from build123d import *

# Parameters (mm, degrees)
BOSS_EXTRUDE1_DEPTH = 45
SKETCH4_R           = 1.35
CUT_EXTRUDE3_DEPTH  = 88.759301296
SKETCH16_W          = 54.601375451
SKETCH16_H          = 80.563035577
CUT_EXTRUDE6_DEPTH  = 86.719849393
SKETCH17_W          = 45
SKETCH17_H          = 36.75
SKETCH17_W_2        = 30
SKETCH17_H_2        = 30
CUT_EXTRUDE7_DEPTH  = 74.310606081
SKETCH18_R          = 1.35
CUT_EXTRUDE8_DEPTH  = 64.93499752
FILLET1_R           = 8.89
SKETCH19_W          = 11
SKETCH19_H          = 11
BOSS_EXTRUDE2_DEPTH = 2.921
SKETCH20_W          = 5
SKETCH20_H          = 5
CUT_EXTRUDE9_DEPTH  = 25
SKETCH26_W          = 32.004
SKETCH26_H          = 43.2054
BOSS_EXTRUDE3_DEPTH = 2.54
SKETCH27_W          = 32.004
SKETCH27_H          = 22.606
BOSS_EXTRUDE4_DEPTH = 11.7475
SKETCH28_R          = 1.2954
CUT_EXTRUDE11_DEPTH = 19.05
CUT_EXTRUDE14_DEPTH = 3.81
SKETCH32_W          = 2.921
SKETCH32_H          = 9.5
BOSS_EXTRUDE5_DEPTH = 10.922
SKETCH33_W          = 11.7475
SKETCH33_H          = 20.574
CUT_EXTRUDE15_DEPTH = 78.55193447
FILLET2_R           = 5.08
FILLET3_R           = 5.08
FILLET4_R           = 7.62
FILLET5_R           = 7.62
FILLET6_R           = 7.62
FILLET7_R           = 2.54
FILLET8_R           = 2.54
FILLET9_R           = 2.54
FILLET10_R          = 2.54
CUT_EXTRUDE16_START = -11.43
SKETCH34_R          = 1.35
CUT_EXTRUDE16_DEPTH = 11.43


with BuildPart() as part:
    # Sketch1 → Boss-Extrude1 (new body)
    with BuildSketch(Plane.XY):
        Polygon((-3.796, -4.492), (-3.796, 57.658), (44.704, 57.658), (44.704, 20.908), (39.704, 20.908), (39.704, 52.658), (1.204, 52.658), (1.204, -4.492), align=None)
    extrude(amount=BOSS_EXTRUDE1_DEPTH)

    # Sketch4 → Cut-Extrude3 (cut, through all)
    with BuildSketch(Plane(origin=(44.704, 0, 0), x_dir=(0, 0, -1), z_dir=(1, 0, 0))):
        with Locations(Location((-22.6336, 47.4432, 0), (0, 0, 90))):
            Circle(SKETCH4_R)
        with Locations(Location((-22.6336, 25.448, 0), (0, 0, 90))):
            Circle(SKETCH4_R)
        with Locations(Location((-11.6341, 36.4435, 0), (0, 0, 90))):
            Circle(SKETCH4_R)
        with Locations(Location((-33.6321, 36.4435, 0), (0, 0, 90))):
            Circle(SKETCH4_R)
    extrude(amount=-CUT_EXTRUDE3_DEPTH, mode=Mode.SUBTRACT)

    # Sketch16 → Cut-Extrude6 (cut, through all)
    with BuildSketch(Plane.XY.offset(45)):
        with Locations((12.403312274, 23.911522997)):
            Rectangle(SKETCH16_W, SKETCH16_H)
    extrude(amount=-CUT_EXTRUDE6_DEPTH, mode=Mode.SUBTRACT)

    # Sketch17 → Cut-Extrude7 (cut, through all)
    with BuildSketch(Plane(origin=(44.704, 0, 0), x_dir=(0, 0, -1), z_dir=(1, 0, 0))):
        with Locations((-22.5, 39.283)):
            Rectangle(SKETCH17_W, SKETCH17_H)
        with Locations((-22.6331, 36.4435)):
            Rectangle(SKETCH17_W_2, SKETCH17_H_2, mode=Mode.SUBTRACT)
    extrude(amount=-CUT_EXTRUDE7_DEPTH, mode=Mode.SUBTRACT)

    # Sketch18 → Cut-Extrude8 (cut, through all)
    with BuildSketch(Plane(origin=(44.704, 0, 0), x_dir=(0, 0, -1), z_dir=(1, 0, 0))):
        with Locations(Location((-14.857193174, 44.222006826, 0), (0, 0, 90))):
            Circle(SKETCH18_R)
        with Locations(Location((-30.410360379, 28.668839621, 0), (0, 0, 90))):
            Circle(SKETCH18_R)
        with Locations(Location((-14.856839621, 28.668839621, 0), (0, 0, 90))):
            Circle(SKETCH18_R)
        with Locations(Location((-30.410360379, 44.222006826, 0), (0, 0, 90))):
            Circle(SKETCH18_R)
    extrude(amount=-CUT_EXTRUDE8_DEPTH, mode=Mode.SUBTRACT)

    # Fillet1
    fillet1_edges = [part.edges().sort_by_distance(p)[0] for p in [
        (42.204, 51.4435, 7.6331),
        (42.204, 51.4435, 37.6331),
        (42.204, 21.4435, 37.6331),
        (42.204, 21.4435, 7.6331),
    ]]
    fillet(fillet1_edges, radius=FILLET1_R)

    # Sketch19 → Boss-Extrude2 (add)
    with BuildSketch(Plane(origin=(44.704, 0, 0), x_dir=(0, 0, -1), z_dir=(1, 0, 0))):
        with Locations((-22.6336, 36.4435)):
            Rectangle(SKETCH19_W, SKETCH19_H)
    extrude(amount=BOSS_EXTRUDE2_DEPTH)

    # Sketch20 → Cut-Extrude9 (cut)
    with BuildSketch(Plane(origin=(47.625, 0, 0), x_dir=(0, 0, -1), z_dir=(1, 0, 0))):
        with Locations((-22.6336, 36.4435)):
            Rectangle(SKETCH20_W, SKETCH20_H)
    extrude(amount=-CUT_EXTRUDE9_DEPTH, mode=Mode.SUBTRACT)

    # Sketch26 → Boss-Extrude3 (add)
    with BuildSketch(Plane(origin=(47.625, 0, 0), x_dir=(0, 0, -1), z_dir=(1, 0, 0))):
        with Locations((-22.6336, 24.202149454)):
            Rectangle(SKETCH26_W, SKETCH26_H)
    extrude(amount=BOSS_EXTRUDE3_DEPTH)

    # Sketch27 → Boss-Extrude4 (add)
    with BuildSketch(Plane(origin=(50.165, 0, 0), x_dir=(0, 0, -1), z_dir=(1, 0, 0))):
        with Locations((-22.6336, 13.902449454)):
            Rectangle(SKETCH27_W, SKETCH27_H)
    extrude(amount=BOSS_EXTRUDE4_DEPTH)

    # Sketch28 → Cut-Extrude11 (cut)
    with BuildSketch(Plane(origin=(61.9125, 0, 0), x_dir=(0, 0, -1), z_dir=(1, 0, 0))):
        with Locations((-9.1208, 21.903449454)):
            Circle(SKETCH28_R)
        with Locations((-9.1208, 5.901449454)):
            Circle(SKETCH28_R)
        with Locations((-36.1464, 5.901449454)):
            Circle(SKETCH28_R)
        with Locations((-36.1464, 21.903449454)):
            Circle(SKETCH28_R)
    extrude(amount=-CUT_EXTRUDE11_DEPTH, mode=Mode.SUBTRACT)

    # Sketch31 → Cut-Extrude14 (cut)
    with BuildSketch(Plane(origin=(50.165, 0, 0), x_dir=(0, 0, -1), z_dir=(1, 0, 0))):
        Polygon((-38.6356, 45.804849454), (-38.6356, 30.9435), (-28.1336, 30.9435), (-28.1336, 41.9435), (-17.1336, 41.9435), (-17.1336, 30.9435), (-6.6316, 30.9435), (-6.6316, 45.804849454), align=None)
    extrude(amount=-CUT_EXTRUDE14_DEPTH, mode=Mode.SUBTRACT)

    # Sketch32 → Boss-Extrude5 (add)
    with BuildSketch(Plane(origin=(0, 0, 17.1336), x_dir=(-1, 0, 0), z_dir=(0, 0, -1))):
        with Locations((-46.1645, 26.1935)):
            Rectangle(SKETCH32_W, SKETCH32_H)
    extrude(amount=-BOSS_EXTRUDE5_DEPTH)

    # Sketch33 → Cut-Extrude15 (cut, through all)
    with BuildSketch(Plane(origin=(0, 25.205449454, 0), x_dir=(1, 0, 0), z_dir=(0, 1, 0))):
        with Locations((56.03875, -22.6336)):
            Rectangle(SKETCH33_W, SKETCH33_H)
    extrude(amount=-CUT_EXTRUDE15_DEPTH, mode=Mode.SUBTRACT)

    # Fillet2
    fillet2_edges = [part.edges().sort_by_distance(p)[0] for p in [
        (50.165, 25.205449454, 35.7781),
    ]]
    fillet(fillet2_edges, radius=FILLET2_R)

    # Fillet3
    fillet3_edges = [part.edges().sort_by_distance(p)[0] for p in [
        (50.165, 25.205449454, 9.4891),
    ]]
    fillet(fillet3_edges, radius=FILLET3_R)

    # Fillet4
    # the kernel refuses this fillet: 7.62 mm, written as the material it adds along each edge
    with BuildSketch(Plane(origin=(47.625, 21.4435, 17.1336), x_dir=(-1, 0, 0), z_dir=(0, 0, 1))) as fillet4_piece_1:
        with BuildLine():
            CenterArc((FILLET4_R, FILLET4_R), FILLET4_R, 180, 90)
            Line((0, FILLET4_R), (0, 0))
            Line((0, 0), (FILLET4_R, 0))
        make_face()
    extrude(amount=10.922)

    # Fillet5
    fillet5_edges = [part.edges().sort_by_distance(p)[0] for p in [
        (48.895, 30.9435, 17.1336),
    ]]
    fillet(fillet5_edges, radius=FILLET5_R)

    # Fillet6
    fillet6_edges = [part.edges().sort_by_distance(p)[0] for p in [
        (48.895, 30.9435, 28.1336),
    ]]
    fillet(fillet6_edges, radius=FILLET6_R)

    # Fillet7
    fillet7_edges = [part.edges().sort_by_distance(p)[0] for p in [
        (47.4345, 41.9435, 28.1336),
    ]]
    fillet(fillet7_edges, radius=FILLET7_R)

    # Fillet8
    fillet8_edges = [part.edges().sort_by_distance(p)[0] for p in [
        (47.4345, 41.9435, 17.1336),
    ]]
    fillet(fillet8_edges, radius=FILLET8_R)

    # Fillet9
    fillet9_edges = [part.edges().sort_by_distance(p)[0] for p in [
        (47.625, 22.3835, 28.0556),
    ]]
    fillet(fillet9_edges, radius=FILLET9_R)

    # Fillet10
    fillet10_edges = [part.edges().sort_by_distance(p)[0] for p in [
        (47.625, 26.1935, 17.1336),
    ]]
    fillet(fillet10_edges, radius=FILLET10_R)

    # Sketch34 → Cut-Extrude16 (cut)
    with BuildSketch(Plane.ZY.offset(-39.704).offset(CUT_EXTRUDE16_START)):
        with Locations(Location((22.6336, 25.448, 0), (0, 0, 90))):
            Circle(SKETCH34_R)
    extrude(amount=CUT_EXTRUDE16_DEPTH, mode=Mode.SUBTRACT)


solid = part.part
Can you work these out from the model? Positions are in its coordinate system, mm. A direction names the side the tool comes from. Give positions to 0.01 mm unless a question says otherwise; leave off trailing zeros. Order: outer loops, then holes, each group sorted by start corner. A loop starts at its lowest first (then second) coordinate and runs counter-clockwise, first axis right, second up. Notation, with made-up numbers: M 79,-34.5 L 85,-34.5 A34 cw 85,1.5 Z; hole C -27,-4 d8. An arc over 180 degrees is marked long. Use one line per item in the form item = value. Start each with the question number.
Item 1: If I drill on line 1 along X through (y, z) = (27, 13) (3 decimals); line 2 along Z through (x, y) = (53.75, 8.5); line 3 along X through (y, z) = (20, 30.5) (3 decimals), over which ranges is the centre line in solid material (lowest first)?
Item 2: If we section it at A-A (x = 57.75): Write out the boundary of the cut face in (y, z), then the cut area to 3 significant figures.
Item 3: For faces 1 (the cylindrical face through (42.24, 35.45, 12.55)), 2 (the flat face through (56, 14, 12.347)), 3 (the flat face through (44, 36, 20.134)), 4 (the cylindrical face through (48.401, 34.124, 29.56)), 5 (the flat face through (59, 25.205, 10)), which set-ups out of +Z, -Z, +X, -X, +Y, -Y let a thin tool reach every point of the face, with its end or its side?
Item 4: Will these pins go through, and if not, where does the flat tip stop? pin 1 Ø2.5 at (y, z) = (5.9, 36.15) entering from -X; pin 2 Ø3.5 at (y, z) = (25.45, 22.63) entering from +X (3 decimals); pin 3 Ø5.5 at (x, z) = (43, 20.5) entering from -Y; pin 4 Ø10 at (x, z) = (49.5, 14) entering from +Y.
Item 5: If we section it at D-D (x = 48.75): Write out the boundary of the cut face in (y, z).
Item 6: If we section it at B-B (y = 36): Write out the boundary of the cut face in (x, z) (3 decimals).
Item 7: We'd pull the mould along Y, two halves only. Please class faces 6 (the cylindrical face through (45.452, 19.152, 22.483)), 7 (the flat face through (39.704, 36.2, 19.5)), 8 (the flat face through (44, 33.944, 23)), 9 (the flat face through (59, 25.205, 36)): +Y half, -Y half, draft (parallel to the pull), parting line (faces both ways), or undercut.
Outcome:
q1.line_1 = 39.704 to 44.704, 47.625 to 50.165
q1.line_2 = 6.63 to 12.35, 32.92 to 38.64
q1.line_3 = 47.623 to 50.165
q2.outline = M 2.6,6.63 L 25.21,6.63 L 25.21,12.35 L 2.6,12.35 Z; M 2.6,32.92 L 25.21,32.92 L 25.21,38.64 L 2.6,38.64 Z; hole C 5.9,9.12 d2.59; hole C 5.9,36.15 d2.59; hole C 21.9,9.12 d2.59; hole C 21.9,36.15 d2.59
q2.area = 237 mm2
q3.face_1 = +X, -X
q3.face_2 = +X, +Y, -Y
q3.face_3 = -X
q3.face_4 = +Z, +X, +Y
q3.face_5 = +Z, -Z, +X, +Y
q4.pin_1 = through
q4.pin_2 = 50.165
q4.pin_3 = 18.83
q4.pin_4 = 51.37
q5.outline = M 2.6,6.63 L 30.94,6.63 L 30.94,9.51 A7.62 cw 38.56,17.13 L 39.4,17.13 A2.54 ccw 41.94,19.67 L 41.94,25.59 A2.54 ccw 39.4,28.13 L 38.56,28.13 A7.62 cw 30.94,35.75 L 30.94,38.64 L 2.6,38.64 Z; hole C 5.9,9.12 d2.59; hole C 5.9,36.15 d2.59; hole C 21.9,9.12 d2.59; hole C 21.9,36.15 d2.59; hole C 25.45,22.63 d2.7
q6.outline = M 39.704,7.633 L 44.704,7.633 L 44.704,10.359 L 39.704,10.359 Z; M 39.704,12.909 L 44.704,12.909 L 44.704,17.134 L 45.085,17.134 A2.54 cw 46.52,16.689 L 50.165,16.689 L 50.165,28.578 L 46.628,28.578 A2.54 cw 45.71,28.134 L 44.704,28.134 L 44.704,32.357 L 39.704,32.357 L 39.704,25.134 L 47.625,25.134 L 47.625,20.134 L 39.704,20.134 Z; M 39.704,34.907 L 44.704,34.907 L 44.704,37.633 L 39.704,37.633 Z
q7.face_6 = -Y half
q7.face_7 = draft
q7.face_8 = undercut
q7.face_9 = +Y half
